```python
from build123d import *

# Parameters (mm, degrees)
BOSS_EXTRUDE1_DEPTH = 10
CUT_EXTRUDE1_REACH  = 29.981
SKETCH3_R           = 5
BOSS_EXTRUDE2_DEPTH = 2
FILLET1_R           = 1
CUT_EXTRUDE2_REACH  = 26.783
SKETCH5_R           = 2
SKETCH6_R           = 3.5
CUT_EXTRUDE3_DEPTH  = 4


with BuildPart() as part:
    # Sketch2 → Boss-Extrude1 (new body)
    with BuildSketch(Plane(origin=(0, 0, 0), x_dir=(0, 0, -1), z_dir=(1, 0, 0))):
        Polygon((0, 0), (12, 0), (12, -7.5), (21.4, -7.5), (21.4, -15), (-9.4, -15), (-9.4, -7.5), (0, -7.5), align=None)
    extrude(amount=BOSS_EXTRUDE1_DEPTH)

    # Sketch3 → Cut-Extrude1 (cut, up to next)
    with BuildSketch(Plane(origin=(10, 0, 0), x_dir=(0, 0, -1), z_dir=(1, 0, 0)), mode=Mode.PRIVATE) as cut_extrude1_sk1:
        with Locations((6, -7)):
            Circle(SKETCH3_R)
    cut_extrude1_tool1 = extrude(cut_extrude1_sk1.sketch, amount=-CUT_EXTRUDE1_REACH, mode=Mode.PRIVATE) & part.part
    add(cut_extrude1_tool1.solids().sort_by_distance((10, -7, -6))[0], mode=Mode.SUBTRACT)

    # Sketch4 → Boss-Extrude2 (add)
    with BuildSketch(Plane.ZY):
        Polygon((0, -7.5), (0, 0), (-12, 0), (-12, -7.5), (-21.4, -7.5), (-21.4, -15), (9.4, -15), (9.4, -7.5), align=None)
    extrude(amount=BOSS_EXTRUDE2_DEPTH)

    # Fillet1
    fillet1_edges = [part.edges().sort_by_distance(p)[0] for p in [
        (4, 0, 0),
        (4, 0, -12),
        (4, -7.5, -12),
        (4, -7.5, 0),
    ]]
    fillet(fillet1_edges, radius=FILLET1_R)

    # Sketch5 → Cut-Extrude2 (cut, up to next)
    with BuildSketch(Plane(origin=(0, -7.5, 0), x_dir=(1, 0, 0), z_dir=(0, 1, 0)), mode=Mode.PRIVATE) as cut_extrude2_sk1:
        with Locations(Location((4, 17.2, 0), (0, 0, 270))):
            Circle(SKETCH5_R)
    cut_extrude2_tool1 = extrude(cut_extrude2_sk1.sketch, amount=-CUT_EXTRUDE2_REACH, mode=Mode.PRIVATE) & part.part
    # Sketch5 → Cut-Extrude2 (cut, up to next)
    with BuildSketch(Plane(origin=(0, -7.5, 0), x_dir=(1, 0, 0), z_dir=(0, 1, 0)), mode=Mode.PRIVATE) as cut_extrude2_sk2:
        with Locations(Location((4, -5.2, 0), (0, 0, 270))):
            Circle(SKETCH5_R)
    cut_extrude2_tool2 = extrude(cut_extrude2_sk2.sketch, amount=-CUT_EXTRUDE2_REACH, mode=Mode.PRIVATE) & part.part
    add(cut_extrude2_tool1.solids().sort_by_distance((4, -7.5, -17.2))[0], mode=Mode.SUBTRACT)
    add(cut_extrude2_tool2.solids().sort_by_distance((4, -7.5, 5.2))[0], mode=Mode.SUBTRACT)

    # Sketch6 → Cut-Extrude3 (cut)
    with BuildSketch(Plane(origin=(0, -7.5, 0), x_dir=(1, 0, 0), z_dir=(0, 1, 0))):
        with Locations(Location((4, -5.2, 0), (0, 0, 270))):
            Circle(SKETCH6_R)
        with Locations(Location((4, 17.2, 0), (0, 0, 270))):
            Circle(SKETCH6_R)
    extrude(amount=-CUT_EXTRUDE3_DEPTH, mode=Mode.SUBTRACT)


solid = part.part
```
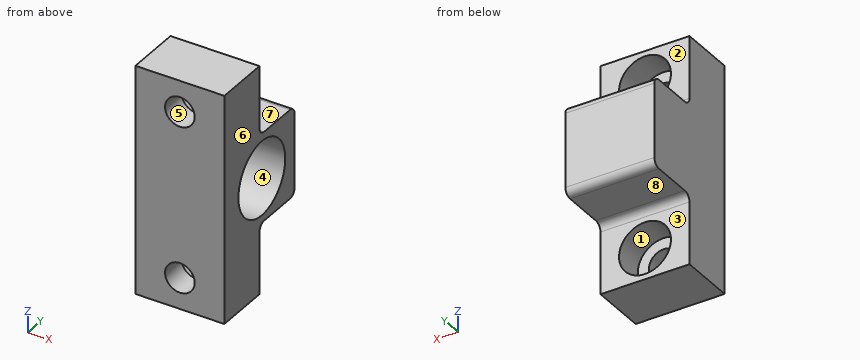
Source: CAD feature listing. Evaluate the final solid. Frame: model axes, mm. Face numbers are marked on the shaded views. A direction names the side the tool comes from. Give positions to 0.01 mm unless a question says otherwise; leave off trailing zeros. Write each loop counter-clockwise with the first axis right and the second up, starting at its lowest first coordinate (ties: lowest second). Pieces come first, ordered by that corner, then holes. Notation, with made-up numbers: (54.25, 71.5) - (88.25, 71.5) arc R26 ccw to (88.25, 93.5) - close; hole circle Ø7 at (44, -26.75). An arc over 180 degrees is marked (long way). One line per item, written item: value. Start each with the question number.
Q1. Draft query along Z for the marked faces 5, 6, 7 and 8. Return one class per face: +Z half, -Z half, draft (parallel to the pull), parting line (faces both ways), or undercut.
Q2. First-contact query: pin 1 Ø6 at (x, y) = (4.5, -3.5) entering from -Z; pin 2 Ø2.5 at (x, z) = (2.5, -16.5) entering from +Y; pin 3 Ø6 at (x, y) = (2, -3.5) entering from +Z; pin 4 Ø6.5 at (x, z) = (4, 5.2) entering from -Y. Flat tips, straight axial feed; report the tip coordinate or a pass-through.
Q3. Set-up query: the marked faces 1, 2, 3 and 4. Return all of +Z, -Z, +X, -X, +Y, -Y with unobstructed straight access to the full face (end or side cutting, diameter ignored); none if empty.
Q4. Section query D-D, the plane x = 8. Return the cut outline in (y, z).
Q5. Section query A-A, the plane x = 4. Count the separate pieces of the cut face and the enclosed holes in it, then the cut area to 3 significant figures.
Q6. Material intervals for probe 1 along X at (y, z) = (-13.4, 5.2); probe 2 along Z at (x, y) = (2.25, -9); probe 3 along Z at (x, y) = (5, -9), sorted ascending. Write a range as from..to.
Q7. Section query B-B, the plane z = 5.2. Return the cut outline in (x, y), then the cut area to 3 significant figures.
Q8. Section query C-C, the plane z = -6. Return the cut outline in (x, y), then the cut area to 3 significant figures.
Answer:
1. face 5: undercut
1. face 6: draft
1. face 7: +Z half
1. face 8: -Z half
2. pin 1: stops at z = -12
2. pin 2: stops at y = -11.5
2. pin 3: stops at z = 0
2. pin 4: stops at y = -15
3. face 1: +Y
3. face 2: +Z, +X, -X, +Y
3. face 3: -Z, +X, -X, +Y
3. face 4: +X
4. outline: (-15, -21.4) - (-7.5, -21.4) - (-7.5, -13) arc R1 cw to (-6.5, -12) - (-1, -12) arc R1 ccw to (0, -11) - (0, -1) arc R1 ccw to (-1, 0) - (-6.5, 0) arc R1 cw to (-7.5, 1) - (-7.5, 9.4) - (-15, 9.4) - close; hole circle Ø10 at (-7, -6)
5. separate pieces: 3
5. enclosed holes: 1
5. area: 158 mm2
6. probe 1: x = -2..2, 6..10
6. probe 2: z = -21.4..-20.23, -14.17..-10.58, -1.42..2.17, 8.23..9.4
6. probe 3: z = -21.4..-20.55, -13.85..-10.58, -1.42..1.85, 8.55..9.4
7. outline: (-2, -15) - (2, -15) - (2, -11.5) - (0.5, -11.5) - (0.5, -7.5) - (-2, -7.5) - close; (6, -15) - (10, -15) - (10, -7.5) - (7.5, -7.5) - (7.5, -11.5) - (6, -11.5) - close
7. area: 48.0 mm2
8. outline: (-2, -15) - (10, -15) - (10, -12) - (0, -12) - (0, -2) - (10, -2) - (10, 0) - (-2, 0) - close
8. area: 80.0 mm2
